from build123d import *

# Parameters (mm, degrees)
CYLINDER_R     = 80
CYLINDER_DEPTH = 10
BOX005_W       = 10
BOX005_H       = 10
BOX005_DEPTH   = 10
BOX003_W       = 20
BOX003_H       = 10
BOX003_DEPTH   = 10
BOX010_W       = 70
BOX010_H       = 10
BOX010_DEPTH   = 10
BOX017_W       = 20
BOX017_H       = 10
BOX017_DEPTH   = 10
BOX001_W       = 10
BOX001_H       = 10
BOX001_DEPTH   = 10
BOX008_W       = 110
BOX008_H       = 10
BOX008_DEPTH   = 10
BOX009_W       = 10
BOX009_H       = 10
BOX009_DEPTH   = 10
BOX011_W       = 10
BOX011_H       = 10
BOX011_DEPTH   = 10
BOX016_W       = 20
BOX016_H       = 10
BOX016_DEPTH   = 10
BOX006_W       = 30
BOX006_H       = 10
BOX006_DEPTH   = 10
BOX013_W       = 10
BOX013_H       = 10
BOX013_DEPTH   = 10
BOX015_W       = 10
BOX015_H       = 10
BOX015_DEPTH   = 10
BOX007_W       = 20
BOX007_H       = 10
BOX007_DEPTH   = 10
BOX012_W       = 10
BOX012_H       = 10
BOX012_DEPTH   = 10
BOX002_W       = 70
BOX002_H       = 10
BOX002_DEPTH   = 10
BOX014_W       = 10
BOX014_H       = 10
BOX014_DEPTH   = 10
BOX004_W       = 10
BOX004_H       = 10
BOX004_DEPTH   = 10
BOX_W          = 10
BOX_H          = 10
BOX_DEPTH      = 10


with BuildPart() as cilindro:
    # Cylinder → Cylinder (new body)
    with BuildSketch(Plane.XY.offset(-10)):
        Circle(CYLINDER_R)
    extrude(amount=CYLINDER_DEPTH)


with BuildPart() as cubo005:
    # Box005 → Box005 (new body)
    with BuildSketch(Plane(origin=(50, -10, 0), x_dir=(1, 0, 0), z_dir=(0, 0, 1))):
        with Locations((5, 5)):
            Rectangle(BOX005_W, BOX005_H)
    extrude(amount=BOX005_DEPTH)


with BuildPart() as cubo003:
    # Box003 → Box003 (new body)
    with BuildSketch(Plane(origin=(-10, -30, 0), x_dir=(1, 0, 0), z_dir=(0, 0, 1))):
        with Locations((10, 5)):
            Rectangle(BOX003_W, BOX003_H)
    extrude(amount=BOX003_DEPTH)


with BuildPart() as cubo010:
    # Box010 → Box010 (new body)
    with BuildSketch(Plane(origin=(0, -50, 0), x_dir=(1, 0, 0), z_dir=(0, 0, 1))):
        with Locations((35, 5)):
            Rectangle(BOX010_W, BOX010_H)
    extrude(amount=BOX010_DEPTH)


with BuildPart() as cubo017:
    # Box017 → Box017 (new body)
    with BuildSketch(Plane(origin=(40, -70, 0), x_dir=(1, 0, 0), z_dir=(0, 0, 1))):
        with Locations((10, 5)):
            Rectangle(BOX017_W, BOX017_H)
    extrude(amount=BOX017_DEPTH)


with BuildPart() as cubo001:
    # Box001 → Box001 (new body)
    with BuildSketch(Plane(origin=(10, -10, 0), x_dir=(1, 0, 0), z_dir=(0, 0, 1))):
        with Locations((5, 5)):
            Rectangle(BOX001_W, BOX001_H)
    extrude(amount=BOX001_DEPTH)


with BuildPart() as cubo008:
    # Box008 → Box008 (new body)
    with BuildSketch(Plane(origin=(-20, -40, 0), x_dir=(1, 0, 0), z_dir=(0, 0, 1))):
        with Locations((55, 5)):
            Rectangle(BOX008_W, BOX008_H)
    extrude(amount=BOX008_DEPTH)


with BuildPart() as cubo009:
    # Box009 → Box009 (new body)
    with BuildSketch(Plane(origin=(-20, -50, 0), x_dir=(1, 0, 0), z_dir=(0, 0, 1))):
        with Locations((5, 5)):
            Rectangle(BOX009_W, BOX009_H)
    extrude(amount=BOX009_DEPTH)


with BuildPart() as cubo011:
    # Box011 → Box011 (new body)
    with BuildSketch(Plane(origin=(80, -50, 0), x_dir=(1, 0, 0), z_dir=(0, 0, 1))):
        with Locations((5, 5)):
            Rectangle(BOX011_W, BOX011_H)
    extrude(amount=BOX011_DEPTH)


with BuildPart() as cubo016:
    # Box016 → Box016 (new body)
    with BuildSketch(Plane(origin=(10, -70, 0), x_dir=(1, 0, 0), z_dir=(0, 0, 1))):
        with Locations((10, 5)):
            Rectangle(BOX016_W, BOX016_H)
    extrude(amount=BOX016_DEPTH)


with BuildPart() as cubo006:
    # Box006 → Box006 (new body)
    with BuildSketch(Plane(origin=(20, -30, 0), x_dir=(1, 0, 0), z_dir=(0, 0, 1))):
        with Locations((15, 5)):
            Rectangle(BOX006_W, BOX006_H)
    extrude(amount=BOX006_DEPTH)


with BuildPart() as cubo013:
    # Box013 → Box013 (new body)
    with BuildSketch(Plane(origin=(0, -60, 0), x_dir=(1, 0, 0), z_dir=(0, 0, 1))):
        with Locations((5, 5)):
            Rectangle(BOX013_W, BOX013_H)
    extrude(amount=BOX013_DEPTH)


with BuildPart() as cubo015:
    # Box015 → Box015 (new body)
    with BuildSketch(Plane(origin=(80, -60, 0), x_dir=(1, 0, 0), z_dir=(0, 0, 1))):
        with Locations((5, 5)):
            Rectangle(BOX015_W, BOX015_H)
    extrude(amount=BOX015_DEPTH)


with BuildPart() as cubo007:
    # Box007 → Box007 (new body)
    with BuildSketch(Plane(origin=(60, -30, 0), x_dir=(1, 0, 0), z_dir=(0, 0, 1))):
        with Locations((10, 5)):
            Rectangle(BOX007_W, BOX007_H)
    extrude(amount=BOX007_DEPTH)


with BuildPart() as cubo012:
    # Box012 → Box012 (new body)
    with BuildSketch(Plane(origin=(-20, -60, 0), x_dir=(1, 0, 0), z_dir=(0, 0, 1))):
        with Locations((5, 5)):
            Rectangle(BOX012_W, BOX012_H)
    extrude(amount=BOX012_DEPTH)


with BuildPart() as cubo002:
    # Box002 → Box002 (new body)
    with BuildSketch(Plane(origin=(0, -20, 0), x_dir=(1, 0, 0), z_dir=(0, 0, 1))):
        with Locations((35, 5)):
            Rectangle(BOX002_W, BOX002_H)
    extrude(amount=BOX002_DEPTH)


with BuildPart() as cubo014:
    # Box014 → Box014 (new body)
    with BuildSketch(Plane(origin=(60, -60, 0), x_dir=(1, 0, 0), z_dir=(0, 0, 1))):
        with Locations((5, 5)):
            Rectangle(BOX014_W, BOX014_H)
    extrude(amount=BOX014_DEPTH)


with BuildPart() as cubo004:
    # Box004 → Box004 (new body)
    with BuildSketch(Plane(origin=(60, 0, 0), x_dir=(1, 0, 0), z_dir=(0, 0, 1))):
        with Locations((5, 5)):
            Rectangle(BOX004_W, BOX004_H)
    extrude(amount=BOX004_DEPTH)


with BuildPart() as fusion001:
    # Box → Box (new body)
    with BuildSketch(Plane.XY):
        with Locations((5, 5)):
            Rectangle(BOX_W, BOX_H)
    extrude(amount=BOX_DEPTH)

    # Fusion: union Cubo005, Cubo003, Cubo010, Cubo017, Cubo001, Cubo008, Cubo009, Cubo011, Cubo016, Cubo006, Cubo013, Cubo015, Cubo007, Cubo012, Cubo002, Cubo014, Cubo004
    add(cubo005.part)
    add(cubo003.part)
    add(cubo010.part)
    add(cubo017.part)
    add(cubo001.part)
    add(cubo008.part)
    add(cubo009.part)
    add(cubo011.part)
    add(cubo016.part)
    add(cubo006.part)
    add(cubo013.part)
    add(cubo015.part)
    add(cubo007.part)
    add(cubo012.part)
    add(cubo002.part)
    add(cubo014.part)
    add(cubo004.part)


with BuildPart() as fusion001_1:
    # Fusion placement: moved
    add(fusion001.part.moved(Location((-35, 30, 0))))

    # Fusion001: union Cilindro
    add(cilindro.part)


solid = fusion001_1.part
The listing builds one solid part. Answer for the finished solid, in the listing's coordinates (mm). A direction names the side the tool comes from. Round coordinates to 2 decimals unless told otherwise and drop trailing zeros. Loops run counter-clockwise (first coordinate to the right, second up) from the corner with the lowest first, then second, coordinate; pieces in that order, holes last. Notation, with made-up numbers: M -10.5,83 L 34.5,83 A14 cw 34.5,108 Z; hole C 33.25,47 d4. An arc over 180 degrees is marked long. Return JSON: item names as keys, results as strings.
Q1. The mould has two halves that part along X. Classify faces 5 (the face through (-15, -35, 10)), 6 (the face through (20, 0, 5)), 7 (the face through (-25, 25, 5)): released by +X, released by -X, zero draft, split by the parting line, or undercut.
Results list:
{"face 5": "zero draft", "face 6": "undercut", "face 7": "released by -X"}
Q2. Which of the six approach directions +Z, -Z, +X, -X, +Y, -Y give full straight-line access (tool end or side, diameter ignored) to faces 1 (the face through (30, 40, 5)), 2 (the face through (25, -25, 5)), 3 (the face through (15, -40, 5)), 4 (the face through (-40, 10, 5))?
Results list:
{"face 1": "+Z, +X, -X, +Y", "face 2": "+Z", "face 3": "+Z, +X, -X, -Y", "face 4": "+Z, -X, +Y"}
Q3. Find section D-D, the plane y = 66.5. Determine the outline of the cut face in (x, z).
Results list:
{"outline": "M -44.47,-10 L 44.47,-10 L 44.47,0 L -44.47,0 Z"}
Q4. Each of these flat-tipped pins is pushed along its axis until it touches: pin 1 Ø8 at (x, z) = (48, 3.5) entering from -Y; pin 2 Ø5 at (x, z) = (38.5, 7) entering from +Y; pin 3 Ø12 at (x, y) = (-30.5, -45) entering from +Z. Where does it stop, or does it pass through?
Results list:
{"pin 1": "stops at y = -65.41", "pin 2": "stops at y = 10", "pin 3": "stops at z = 0"}
Q5. Find section B-B, the plane x = 0. Determine the outline of the cut face in (y, z).
Results list:
{"outline": "M -80,-10 L 80,-10 L 80,0 L 20,0 L 20,10 L -20,10 L -20,0 L -80,0 Z"}
Q6. Find section C-C, the plane z = -4. Determine the outline of the cut face in (x, y).
Results list:
{"outline": "C 0,0 d160"}
Q7. Find the intervals of material crossed by line 1 along X through (y, z) = (7.5, 5.75); line 2 along Y through (x, z) = (19.5, 4); line 3 along X through (y, z) = (38.5, 6.5), in increasing order. Write a range as from..to.
Results list:
{"line 1": "x = -45..-25, -15..15, 25..45", "line 2": "y = -40..-30, -20..0, 10..30", "line 3": "x = -35..-25, 25..35"}
